Geometry: final body of the model. Coordinates: model frame, mm. Give positions to 0.01 mm unless a question says otherwise; leave off trailing zeros. Write each loop counter-clockwise with the first axis right and the second up, starting at its lowest first coordinate (ties: lowest second). Pieces come first, ordered by that corner, then holes.
from build123d import *

# Parameters (mm, degrees)
F2_W     = 40
F2_H     = 10
F3_DEPTH = 12.5
F4_R     = 8
F5_DEPTH = 24.811


with BuildPart() as f1:
    # F0 (on Top) → F1 (revolve)
    with BuildSketch(Plane.XY):
        with BuildLine():
            Line((-14.275, 0), (14.275, 0))
            ThreePointArc((14.275, 0), (0, 14.275), (-14.275, 0))
        make_face()
    revolve(axis=Axis((0, 0, 0), (1, 0, 0)))

    # F2 (on Front) → F3 (cut, symmetric)
    with BuildSketch(Plane.XZ):
        with Locations((0, 15.535)):
            Rectangle(F2_W, F2_H)
        with Locations((0, -15.535)):
            Rectangle(F2_W, F2_H)
    extrude(amount=F3_DEPTH, both=True, mode=Mode.SUBTRACT)

    # F4 (on face) → F5 (cut, through all)
    with BuildSketch(Plane.XY.offset(10.535)):
        Circle(F4_R)
    extrude(amount=-F5_DEPTH, mode=Mode.SUBTRACT)


solid = f1.part
Q1. Pin query (flat end, axial travel): P1, Ø2, axis at x = 9.5, y = 7.5, coming from the -Z side; P2, Ø5, axis at y = -8, z = 10, coming from the -X side; P3, Ø5, axis at y = -6, z = 2, coming from the +X side. Return the tip coordinate at first contact, or that it passes through.
Filled sheet:
P1: stops at z = -8.97
P2: stops at x = -9.88
P3: stops at x = 13.75
Q2. Section A-A on y = 0. Output: boundary loops of the cut face in (x, z) (3 decimals).
Filled sheet:
outline: (-9.633, -10.535) - (-8, -10.535) - (-8, 10.535) - (-9.633, 10.535) arc R14.275 ccw to start; (8, -10.535) - (9.633, -10.535) arc R14.275 ccw to (9.633, 10.535) - (8, 10.535) - close
Q3. Section C-C on z = -6. Output: boundary loops of the cut face in (x, y).
Filled sheet:
outline: circle Ø25.91 at (0, 0); hole circle Ø16 at (0, 0)
Q4. Section D-D on x = -12.25. Output: boundary loops of the cut face in (y, z), plus the area to 3 significant figures.
Filled sheet:
outline: circle Ø14.66 at (0, 0)
area: 169 mm2
Q5. Pull-direction query (Y, two-part tool) for faces 1 (the flat face through (-2, -8, -10.535)), 2 (the cylindrical face through (-1.73, -7.81, 0.15)); classes: released by +Y, released by -Y, zero draft, split by the parting line, or undercut.
Filled sheet:
face 1: zero draft
face 2: undercut
Q6. Ray query, line 1 along Y through (x, z) = (0, -0.5); line 2 along Z through (x, y) = (-1.25, -8) (3 decimals); line 3 along Y through (x, z) = (0.25, -2.5). Return the intervals inside material, ascending.
Filled sheet:
line 1: y = -14.27 to -8, 8 to 14.27
line 2: z = -10.535 to 10.535
line 3: y = -14.05 to -8, 8 to 14.05
